```python
from build123d import *

# Parameters (mm, degrees)
SKETCH3_R           = 1.3499999999999943
SKETCH3_R_2         = 1.6999999999999862
SKETCH3_R_3         = 1.699999999999979
SKETCH3_R_4         = 1.699999999999964
SKETCH3_R_5         = 1.3500000000000039
BOSS_EXTRUDE2_DEPTH = 2.54
BOSS_EXTRUDE3_START = -3.175
SKETCH3_3_R         = 1.6999999999999862
SKETCH3_3_R_2       = 3.174999999999997
SKETCH3_3_R_3       = 1.699999999999979
SKETCH3_3_R_4       = 3.174999999999995
SKETCH3_3_R_5       = 1.699999999999964
SKETCH3_3_R_6       = 3.174999999999986
BOSS_EXTRUDE3_DEPTH = 3.175
SKETCH3_4_R         = 3.174999999999997
BOSS_EXTRUDE4_DEPTH = 6.35


with BuildPart() as part:
    # Sketch3 → Boss-Extrude2 (new body)
    with BuildSketch(Plane(origin=(0, 0, 0), x_dir=(1, 0, 0), z_dir=(0, 1, 0))):
        with BuildLine():
            Line((96.19599726769601, -106.66012454600286), (100.36189241194512, -106.66012454600286))
            Line((100.36189241194512, -106.66012454600286), (100.36189241194512, -115.36017299280766))
            ThreePointArc((100.36189241194512, -115.36017299280765), (98.1168283816778, -120.78023702307492), (103.5368924119451, -118.53517299280766))
            Line((103.53689241194512, -118.53517299280766), (155.1868924119451, -118.53517299280766))
            ThreePointArc((155.1868924119451, -118.53517299280766), (160.6069564422124, -120.78023702307495), (158.36189241194512, -115.36017299280765))
            Line((158.36189241194512, -115.36017299280766), (158.36189241194512, -106.66012454600286))
            Line((158.36189241194512, -106.66012454600286), (174.93599975241602, -106.66012454600286))
            ThreePointArc((174.93599975241602, -106.66012454600286), (180.3560637826833, -108.90518857627016), (178.110999752416, -103.4851245460029))
            Line((178.110999752416, -103.48512454600288), (178.110999752416, -65.39612389231417))
            ThreePointArc((178.110999752416, -65.39612389231418), (180.35176956864325, -59.97388277721503), (174.93388802280236, -62.22517299280775))
            Line((174.93388802280236, -62.22517299280775), (96.19388553808236, -62.22517299280775))
            ThreePointArc((96.19388553808236, -62.22517299280775), (90.7738215078151, -59.98010896254048), (93.01888553808237, -65.40017299280773))
            Line((93.01888553808237, -65.40017299280773), (93.01888553808237, -103.48917364649644))
            ThreePointArc((93.01888553808237, -103.48917364649643), (90.77668346464112, -108.90998437006675), (96.19599984872292, -106.6641729425106))
            Line((96.19599984872293, -106.6641729425106), (96.1959998451294, -106.66402188293941))
            ThreePointArc((96.19599984512938, -106.66402188293941), (96.19599915441427, -106.66207321407566), (96.195997267696, -106.66012454600286))
        make_face()
        with Locations(Location((100.36189241194515, -118.53517299280766, 0), (0, 0, 270))):
            Circle(SKETCH3_R, mode=Mode.SUBTRACT)
        with Locations(Location((93.02099984872295, -106.6641729425106, 0), (0, 0, 270))):
            Circle(SKETCH3_R_2, mode=Mode.SUBTRACT)
        with Locations(Location((158.36189241194515, -118.53517299280767, 0), (0, 0, 270))):
            Circle(SKETCH3_R, mode=Mode.SUBTRACT)
        with Locations(Location((93.01888553808237, -62.22517299280775, 0), (0, 0, 270))):
            Circle(SKETCH3_R_3, mode=Mode.SUBTRACT)
        with Locations(Location((178.10888544177544, -62.2211245963, 0), (0, 0, 270))):
            Circle(SKETCH3_R_4, mode=Mode.SUBTRACT)
        with Locations(Location((178.110999752416, -106.66012454600286, 0), (0, 0, 270))):
            Circle(SKETCH3_R_4, mode=Mode.SUBTRACT)
        with Locations(Location((100.36189241194512, -69.53517299280766, 0), (0, 0, 270))):
            Circle(SKETCH3_R_5, mode=Mode.SUBTRACT)
        with Locations(Location((158.36189241194512, -69.53517299280766, 0), (0, 0, 270))):
            Circle(SKETCH3_R, mode=Mode.SUBTRACT)
    extrude(amount=BOSS_EXTRUDE2_DEPTH)

    # Sketch3_3 → Boss-Extrude3 (add)
    # profile 1 of 4: a face of its own
    with BuildSketch(Plane(origin=(0, 0, 0), x_dir=(1, 0, 0), z_dir=(0, 1, 0)).offset(BOSS_EXTRUDE3_START)):
        with BuildLine():
            ThreePointArc((96.19599984512938, -106.66402188293941), (89.84599984962134, -106.6642484722962), (96.19599984872292, -106.6641729425106))
            Line((96.19599984872293, -106.6641729425106), (96.1959998451294, -106.66402188293941))
        make_face()
        with Locations(Location((93.02099984872295, -106.6641729425106, 0), (0, 0, 270))):
            Circle(SKETCH3_3_R, mode=Mode.SUBTRACT)
    # profile 2 of 4: a face of its own
    with BuildSketch(Plane(origin=(0, 0, 0), x_dir=(1, 0, 0), z_dir=(0, 1, 0)).offset(BOSS_EXTRUDE3_START)):
        with Locations(Location((93.01888553808236, -62.22517299280773, 0), (0, 0, 270))):
            Circle(SKETCH3_3_R_2)
        with Locations(Location((93.01888553808237, -62.22517299280775, 0), (0, 0, 270))):
            Circle(SKETCH3_3_R_3, mode=Mode.SUBTRACT)
    # profile 3 of 4: a face of its own
    with BuildSketch(Plane(origin=(0, 0, 0), x_dir=(1, 0, 0), z_dir=(0, 1, 0)).offset(BOSS_EXTRUDE3_START)):
        with Locations(Location((178.10888544177544, -62.22112459630001, 0), (0, 0, 180.073057038))):
            Circle(SKETCH3_3_R_4)
        with Locations(Location((178.10888544177544, -62.2211245963, 0), (0, 0, 270))):
            Circle(SKETCH3_3_R_5, mode=Mode.SUBTRACT)
    # profile 4 of 4: a face of its own
    with BuildSketch(Plane(origin=(0, 0, 0), x_dir=(1, 0, 0), z_dir=(0, 1, 0)).offset(BOSS_EXTRUDE3_START)):
        with Locations(Location((178.110999752416, -106.66012454600288, 0), (0, 0, 90))):
            Circle(SKETCH3_3_R_6)
        with Locations(Location((178.110999752416, -106.66012454600286, 0), (0, 0, 270))):
            Circle(SKETCH3_3_R_5, mode=Mode.SUBTRACT)
    extrude(amount=BOSS_EXTRUDE3_DEPTH)

    # Sketch3_4 → Boss-Extrude4 (add)
    # profile 1 of 4: a face of its own
    with BuildSketch(Plane(origin=(0, 0, 0), x_dir=(1, 0, 0), z_dir=(0, 1, 0))):
        with BuildLine():
            ThreePointArc((100.36189241194512, -115.36017299280766), (102.60695644221241, -116.29010896254037), (103.53689241194512, -118.53517299280766))
            ThreePointArc((103.53689241194512, -118.53517299280766), (98.11682838167783, -120.78023702307495), (100.36189241194512, -115.36017299280766))
        make_face()
        with BuildLine():
            ThreePointArc((100.36189241194512, -117.18517299280768), (99.01189241194514, -118.53517299280766), (100.36189241194512, -119.88517299280767))
            ThreePointArc((100.36189241194512, -119.88517299280767), (101.71189241194513, -118.53517299280766), (100.36189241194512, -117.18517299280768))
        make_face(mode=Mode.SUBTRACT)
    # profile 2 of 4: a face of its own
    with BuildSketch(Plane(origin=(0, 0, 0), x_dir=(1, 0, 0), z_dir=(0, 1, 0))):
        with Locations(Location((100.36189241194512, -69.53517299280767, 0), (0, 0, 270))):
            Circle(SKETCH3_4_R)
        with BuildLine():
            ThreePointArc((100.36189241194512, -68.18517299280767), (99.01189241194511, -69.53517299280767), (100.36189241194512, -70.88517299280767))
            ThreePointArc((100.36189241194512, -70.88517299280767), (101.71189241194512, -69.53517299280767), (100.36189241194512, -68.18517299280767))
        make_face(mode=Mode.SUBTRACT)
    # profile 3 of 4: a face of its own
    with BuildSketch(Plane(origin=(0, 0, 0), x_dir=(1, 0, 0), z_dir=(0, 1, 0))):
        with Locations(Location((158.36189241194512, -69.53517299280767, 0), (0, 0, 270))):
            Circle(SKETCH3_4_R)
        with BuildLine():
            ThreePointArc((158.36189241194512, -68.18517299280767), (157.0118924119451, -69.53517299280767), (158.36189241194512, -70.88517299280767))
            ThreePointArc((158.36189241194512, -70.88517299280767), (159.71189241194512, -69.53517299280767), (158.36189241194512, -68.18517299280767))
        make_face(mode=Mode.SUBTRACT)
    # profile 4 of 4: a face of its own
    with BuildSketch(Plane(origin=(0, 0, 0), x_dir=(1, 0, 0), z_dir=(0, 1, 0))):
        with BuildLine():
            ThreePointArc((155.1868924119451, -118.53517299280766), (160.6069564422124, -120.78023702307496), (158.36189241194512, -115.36017299280766))
            ThreePointArc((158.36189241194512, -115.36017299280766), (156.11682838167783, -116.29010896254037), (155.1868924119451, -118.53517299280766))
        make_face()
        with BuildLine():
            ThreePointArc((158.36189241194512, -117.18517299280768), (157.01189241194515, -118.53517299280766), (158.36189241194512, -119.88517299280767))
            ThreePointArc((158.36189241194512, -119.88517299280767), (159.71189241194514, -118.53517299280766), (158.36189241194512, -117.18517299280768))
        make_face(mode=Mode.SUBTRACT)
    extrude(amount=BOSS_EXTRUDE4_DEPTH)


solid = part.part
```
Verification items for the finished model (mm, model axes). A direction names the side the tool comes from. Coordinates: 2 decimals unless noted, no trailing zeros. Write each loop counter-clockwise with the first axis right and the second up, starting at its lowest first coordinate (ties: lowest second). Pieces come first, ordered by that corner, then holes. Notation, with made-up numbers: M -21.75,38.5 L 5.25,38.5 A32 cw 5.25,68.5 Z; hole C -20.75,-15 d9. An arc over 180 degrees is marked long. Answer as a JSON object with one key per item and string values. Group by question number.
(1) Cross-section at C-C, the plane x = 141.5. Record the cut outline in (y, z), and give its area (3 significant figures).
(2) Tool access check on faces 4 (the face through (180.63, -0.36, 60.29)), 5 (the face through (158.362, 1, 111)), 6 (the face through (129, 1, 118.535)). Record the directions out of +Z, -Z, +X, -X, +Y, -Y that give a thin tool (end or side, any length) a straight path to the whole face; none if there is none.
(3) Material ranges on line 1 (Z direction, x = 178, y = -1); line 2 (Y direction, x = 162, z = 65.5); line 3 (X direction, y = 1.25, z = 94.5), recorded low to high.
(4) Cross-section at A-A, the plane y = 4. Record the cut outline in (x, z) (3 decimals).
(5) Release check for a two-part mould opening along X. For faces 1 (the face through (100, 6.35, 120)), 2 (the face through (155.26, 4.42, 68.85)), 3 (the face through (93.019, 1, 84)) record: +X half, -X half, draft (parallel to the pull), parting line (faces both ways), or undercut.
(6) Gauge pin test, flat ends, axial feed: pin 1 (2.5 mm diameter, centred on x = 93.02, z = 62.23, fed in from +Y); pin 2 (2 mm diameter, centred on x = 104, z = 91, fed in from +Y); pin 3 (5 mm diameter, centred on x = 114.5, y = -1, fed in from +Z); pin 4 (12 mm diameter, centred on x = 106, z = 89, fed in from -Y). Record the tip position at first contact, or that the pin passes through.
(7) Cross-section at B-B, the plane z = 85.5. Record the cut outline in (x, y).
Reply:
{
 "1": {"outline": "M 0,62.23 L 2.54,62.23 L 2.54,118.54 L 0,118.54 Z", "area": "143 mm²"},
 "2": {"face 4": "-Y", "face 5": "+Y, -Y", "face 6": "+Z, +Y, -Y"},
 "3": {"line 1": "59.05 to 60.52, 63.92 to 65.39, 103.49 to 104.96, 108.36 to 109.83", "line 2": "0 to 2.54", "line 3": "93.02 to 178.11"},
 "4": {"outline": "C 100.362,69.535 d6.35; C 100.362,118.535 d6.35; C 158.362,69.535 d6.35; C 158.362,118.535 d6.35; hole C 100.362,69.535 d2.7; hole C 100.362,118.535 d2.7; hole C 158.362,69.535 d2.7; hole C 158.362,118.535 d2.7"},
 "5": {"face 1": "draft", "face 2": "undercut", "face 3": "-X half"},
 "6": {"pin 1": "through", "pin 2": "y = 2.54", "pin 3": "z = 118.54", "pin 4": "y = 0"},
 "7": {"outline": "M 93.02,0 L 178.11,0 L 178.11,2.54 L 93.02,2.54 Z"}
}
